```python
from build123d import *

# Parameters (mm, degrees)
SKETCH1_W           = 55
SKETCH1_H           = 40
BOSS_EXTRUDE1_DEPTH = 40
SKETCH2_R           = 1.6
BOSS_EXTRUDE2_DEPTH = 3.2
BOSS_EXTRUDE3_START = 3.2
SKETCH3_R           = 1.6
BOSS_EXTRUDE3_DEPTH = 3.2
FILLET2_R           = 5
FILLET3_R           = 5
FILLET4_R           = 5
FILLET5_R           = 5


with BuildPart() as part:
    # Sketch1 → Boss-Extrude1 (new body)
    with BuildSketch(Plane.XY):
        Rectangle(SKETCH1_W, SKETCH1_H)
    extrude(amount=BOSS_EXTRUDE1_DEPTH)

    # Sketch2 → Boss-Extrude2 (add)
    with BuildSketch(Plane(origin=(0, 20, 0), x_dir=(1, 0, 0), z_dir=(0, 1, 0))):
        with Locations(Location((-17.5, -20, 0), (0, 0, 90))):
            Circle(SKETCH2_R)
        with Locations(Location((17.5, -20, 0), (0, 0, 90))):
            Circle(SKETCH2_R)
    extrude(amount=BOSS_EXTRUDE2_DEPTH)

    # Sketch3 → Boss-Extrude3 (add)
    with BuildSketch(Plane.XZ.offset(20).offset(BOSS_EXTRUDE3_START)):
        with Locations(Location((-17.5, 20, 0), (0, 0, 270))):
            Circle(SKETCH3_R)
        with Locations(Location((17.5, 20, 0), (0, 0, 270))):
            Circle(SKETCH3_R)
    extrude(amount=-BOSS_EXTRUDE3_DEPTH)

    # Fillet2
    fillet2_edges = [part.edges().sort_by_distance(p)[0] for p in [
        (-27.5, -20, 20),
        (-27.5, 20, 20),
    ]]
    fillet(fillet2_edges, radius=FILLET2_R)

    # Fillet3
    fillet3_edges = [part.edges().sort_by_distance(p)[0] for p in [
        (27.5, -20, 20),
        (27.5, 20, 20),
    ]]
    fillet(fillet3_edges, radius=FILLET3_R)

    # Fillet4
    fillet4_edges = [part.edges().sort_by_distance(p)[0] for p in [
        (0, -20, 40),
        (-27.5, 0, 40),
        (-26.035533906, 18.535533906, 40),
        (-26.035533906, -18.535533906, 40),
        (27.5, 0, 40),
        (0, 20, 40),
        (26.035533906, 18.535533906, 40),
        (26.035533906, -18.535533906, 40),
    ]]
    fillet(fillet4_edges, radius=FILLET4_R)

    # Fillet5
    fillet5_edges = [part.edges().sort_by_distance(p)[0] for p in [
        (0, -20, 0),
        (-27.5, 0, 0),
        (-26.035533906, 18.535533906, 0),
        (-26.035533906, -18.535533906, 0),
        (27.5, 0, 0),
        (0, 20, 0),
        (26.035533906, 18.535533906, 0),
        (26.035533906, -18.535533906, 0),
    ]]
    fillet(fillet5_edges, radius=FILLET5_R)


solid = part.part
```
The model under review builds one solid part; all positions refer to its coordinate system, in mm. A direction names the side the tool comes from. Round coordinates to 2 decimals unless told otherwise and drop trailing zeros. Write each loop counter-clockwise with the first axis right and the second up, starting at its lowest first coordinate (ties: lowest second). Pieces come first, ordered by that corner, then holes. Notation, with made-up numbers: (-16, -19) - (16, -19) arc R25 cw to (16, 2) - close; hole circle Ø8 at (83.5, 26.5). An arc over 180 degrees is marked (long way). One line per question, with ' | ' between items.
Item 1: Add section D-D, the plane x = -11. Give the boundary of the cut face in (y, z).
Resolved:
outline: (-20, 5) arc R5 ccw to (-15, 0) - (15, 0) arc R5 ccw to (20, 5) - (20, 35) arc R5 ccw to (15, 40) - (-15, 40) arc R5 ccw to (-20, 35) - close
Item 2: For faces 1 (the face through (-15.914, -21.622, 20.208)), 2 (the face through (-19.086, 21.578, 20.208)), 3 (the face through (-26.07, -0.21, 1.5)), list the 3-axis set-ups (+Z, -Z, +X, -X, +Y, -Y) from which the entire face can be reached by the end or side of a thin tool; tool diameter is ignored.
Resolved:
face 1: -Y | face 2: +Y | face 3: -Z, -X, +Y, -Y
Item 3: To check wall thickness, follow probe 1 along Y at (x, z) = (-12, 34); probe 2 along X at (y, z) = (19, 3); probe 3 along Z at (x, y) = (22, 19). State the ranges of each line that lie inside material, in increasing order.
Resolved:
probe 1: y = -20 to 20 | probe 2: x = -24.74 to 24.74 | probe 3: z = 2 to 38
Item 4: Add section B-B, the plane x = 17.5. Give the boundary of the cut face in (y, z), then the cut area to 3 significant figures.
Resolved:
outline: (-23.2, 18.4) - (-20, 18.4) - (-20, 5) arc R5 ccw to (-15, 0) - (15, 0) arc R5 ccw to (20, 5) - (20, 18.4) - (23.2, 18.4) - (23.2, 21.6) - (20, 21.6) - (20, 35) arc R5 ccw to (15, 40) - (-15, 40) arc R5 ccw to (-20, 35) - (-20, 21.6) - (-23.2, 21.6) - close | area: 1,600 mm2
Item 5: Add section C-C, the plane z = 11. Give the boundary of the cut face in (x, y), then the cut area to 3 significant figures.
Resolved:
outline: (-27.5, -15) arc R5 ccw to (-22.5, -20) - (22.5, -20) arc R5 ccw to (27.5, -15) - (27.5, 15) arc R5 ccw to (22.5, 20) - (-22.5, 20) arc R5 ccw to (-27.5, 15) - close | area: 2,180 mm2
Item 6: For P1, Ø1.5, axis at x = -2, z = 15, coming from the +Y side; P2, Ø1.5, axis at y = 2.5, z = 36, coming from the +X side; P3, Ø1.5, axis at x = 11.5, z = 15.5, coming from the -Y side, all flat-tipped, find the tip position at first contact; note any pin that passes through.
Resolved:
P1: stops at y = 20 | P2: stops at x = 27.49 | P3: stops at y = -20
Item 7: The part is to be moulded in two halves that separate along X. For faces 4 (the face through (-17, -23.2, 20)), 5 (the face through (-26.07, -0.21, 38.5)), 6 (the face through (19.086, -21.622, 20.208)), say which applies: pulls with the +X half, pulls with the -X half, needs draft (parallel to the pull), parting line crosses it, or undercut.
Resolved:
face 4: needs draft | face 5: pulls with the -X half | face 6: undercut
Item 8: Add section A-A, the plane z = 20. Give the boundary of the cut face in (x, y), then the cut area to 3 significant figures.
Resolved:
outline: (-27.5, -15) arc R5 ccw to (-22.5, -20) - (-19.1, -20) - (-19.1, -23.2) - (-15.9, -23.2) - (-15.9, -20) - (15.9, -20) - (15.9, -23.2) - (19.1, -23.2) - (19.1, -20) - (22.5, -20) arc R5 ccw to (27.5, -15) - (27.5, 15) arc R5 ccw to (22.5, 20) - (19.1, 20) - (19.1, 23.2) - (15.9, 23.2) - (15.9, 20) - (-15.9, 20) - (-15.9, 23.2) - (-19.1, 23.2) - (-19.1, 20) - (-22.5, 20) arc R5 ccw to (-27.5, 15) - close | area: 2,220 mm2
